Work out the finished part from the listing and answer in its coordinate system (mm). Round coordinates to 2 decimals unless told otherwise and drop trailing zeros. Write each loop counter-clockwise with the first axis right and the second up, starting at its lowest first coordinate (ties: lowest second). Pieces come first, ordered by that corner, then holes. Notation, with made-up numbers: M -16.5,-11 L -11.5,-11 A17 cw -11.5,19 Z; hole C -5,72 d1. An arc over 180 degrees is marked long. One line per item, written item: value. Start each with the question number.
Q1. Given pin 1 Ø1.5 at (x, z) = (54, 1) entering from -Y, flat-ended and moving along its own axis, determine where the tip first touches the part or whether it passes through.
Q2. Consider probe 1 along Z at (x, y) = (9.5, 18); probe 2 along X at (y, z) = (64, 5.25). Determine where each line is inside the solid, lowest interval first.
Q3. Find section B-B (z = 3.5). Write down the section's boundary in (x, y).
Q4. Find section C-C (y = 30.5). Write down the section's boundary in (x, z), and give its area (3 significant figures).
Q5. The mould has two halves that part along X. Classify faces 1 (the flat face through (0, 35, 4)), 2 (the cylindrical face through (88.408, 34.609, 2.899)), 3 (the flat face through (49, 70.2, 4)): released by +X, released by -X, zero draft, split by the parting line, or undercut.
Q6. Find section A-A (x = 86.5). Write down the section's boundary in (y, z), and give its area (3 significant figures).
from build123d import *

# Parameters (mm, degrees)
CYLINDER_R       = 2
CYLINDER_DEPTH   = 100
ARRAY002_X_COUNT = 2
ARRAY002_X_PITCH = 77
BOX004_W         = 100
BOX004_H         = 70.2
BOX004_DEPTH     = 9


with BuildPart() as obj1:
    # Cylinder → Cylinder (new body)
    with BuildSketch(Plane(origin=(9.5, -16, 3.5), x_dir=(1, 0, 0), z_dir=(0, 1, 0))):
        Circle(CYLINDER_R)
    extrude(amount=CYLINDER_DEPTH)

    # Array002 X: obj1 ×2


with BuildPart() as obj1_1:
    add(obj1.part)
    with Locations(*[(i * ARRAY002_X_PITCH, 0, 0) for i in range(1, ARRAY002_X_COUNT)]):
        add(obj1.part)


with BuildPart() as obj2:
    # Box004 → Box004 (new body)
    with BuildSketch(Plane.XY):
        with Locations((50, 35.1)):
            Rectangle(BOX004_W, BOX004_H)
    extrude(amount=BOX004_DEPTH)

    # Cut003: cut obj1
    add(obj1_1.part, mode=Mode.SUBTRACT)


solid = obj2.part
The answers:
1. pin 1: y = 0
2. probe 1: 0 to 1.5, 5.5 to 9
2. probe 2: 0 to 8.53, 10.47 to 85.53, 87.47 to 100
3. outline: M 0,0 L 7.5,0 L 7.5,70.2 L 0,70.2 Z; M 11.5,0 L 84.5,0 L 84.5,70.2 L 11.5,70.2 Z; M 88.5,0 L 100,0 L 100,70.2 L 88.5,70.2 Z
4. outline: M 0,0 L 100,0 L 100,9 L 0,9 Z; hole C 9.5,3.5 d4; hole C 86.5,3.5 d4
4. area: 875 mm2
5. face 1: released by -X
5. face 2: undercut
5. face 3: zero draft
6. outline: M 0,0 L 70.2,0 L 70.2,1.5 L 0,1.5 Z; M 0,5.5 L 70.2,5.5 L 70.2,9 L 0,9 Z
6. area: 351 mm2
